Build history of the part. All positions in model axes, mm. Face numbers are marked on the shaded views. A direction names the side the tool comes from. Round coordinates to 2 decimals unless told otherwise and drop trailing zeros. Order: outer loops, then holes, each group sorted by start corner. A loop starts at its lowest first (then second) coordinate and runs counter-clockwise, first axis right, second up. Notation, with made-up numbers: (-14.75, -37) - (30.25, -37) arc R13 cw to (30.25, -14) - close; hole circle Ø8 at (74, 75.5). An arc over 180 degrees is marked (long way). Write each question's results on one line, items separated by ' | '. Start each with the question number.
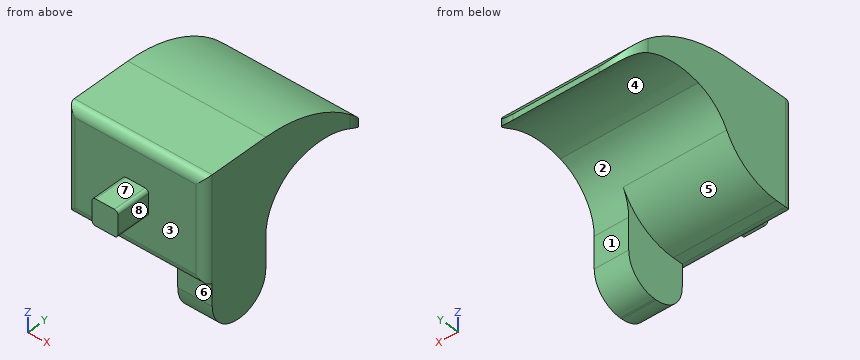
```python
from build123d import *

# Parameters (mm, degrees)
SKETCH1_W           = 80
SKETCH1_H           = 60
BOSS_EXTRUDE1_DEPTH = 40
SKETCH2_W           = 80
SKETCH2_H           = 40
BOSS_EXTRUDE2_DEPTH = 70
CUT_EXTRUDE1_REACH  = 141.284
FILLET4_R           = 31
FILLET6_R           = 5
FILLET7_R           = 15
SKETCH5_W           = 20
SKETCH5_H           = 35
BOSS_EXTRUDE4_DEPTH = 30
FILLET8_R           = 17
FILLET9_R           = 37
SKETCH6_W           = 15
SKETCH6_H           = 15
BOSS_EXTRUDE5_DEPTH = 20
FILLET10_R          = 2


with BuildPart() as part:
    # Sketch1 → Boss-Extrude1 (new body)
    with BuildSketch(Plane(origin=(0, 0, 0), x_dir=(1, 0, 0), z_dir=(0, 1, 0))):
        Rectangle(SKETCH1_W, SKETCH1_H)
    extrude(amount=BOSS_EXTRUDE1_DEPTH)

    # Sketch2 → Boss-Extrude2 (add)
    with BuildSketch(Plane(origin=(0, 40, 0), x_dir=(1, 0, 0), z_dir=(0, 1, 0))):
        with Locations((0, -10)):
            Rectangle(SKETCH2_W, SKETCH2_H)
    extrude(amount=BOSS_EXTRUDE2_DEPTH)

    # Sketch3 → Cut-Extrude1 (cut, up to next)
    with BuildSketch(Plane(origin=(40, 0, 0), x_dir=(0, 0, -1), z_dir=(1, 0, 0)), mode=Mode.PRIVATE) as cut_extrude1_sk1:
        with BuildLine():
            ThreePointArc((10, 110), (-6.715728753, 75), (10, 40))
            Line((10, 40), (10, 110))
        make_face()
    cut_extrude1_tool1 = extrude(cut_extrude1_sk1.sketch, amount=-CUT_EXTRUDE1_REACH, mode=Mode.PRIVATE) & part.part
    # Sketch3 → Cut-Extrude1 (cut, up to next)
    with BuildSketch(Plane(origin=(40, 0, 0), x_dir=(0, 0, -1), z_dir=(1, 0, 0)), mode=Mode.PRIVATE) as cut_extrude1_sk2:
        with BuildLine():
            ThreePointArc((-30, 40), (-20.28517386, 79.505502482), (6.643401936, 110))
            Line((6.643401936, 110), (-30, 110))
            Line((-30, 110), (-30, 40))
        make_face()
    cut_extrude1_tool2 = extrude(cut_extrude1_sk2.sketch, amount=-CUT_EXTRUDE1_REACH, mode=Mode.PRIVATE) & part.part
    add(cut_extrude1_tool1.solids().sort_by_distance((40, 75, -3.194337))[0], mode=Mode.SUBTRACT)
    add(cut_extrude1_tool2.solids().sort_by_distance((40, 93.341036, 19.578223))[0], mode=Mode.SUBTRACT)

    # Fillet4
    fillet4_edges = [part.edges().sort_by_distance(p)[0] for p in [
        (0, 40, -10),
    ]]
    fillet(fillet4_edges, radius=FILLET4_R)

    # Fillet6
    fillet6_edges = [part.edges().sort_by_distance(p)[0] for p in [
        (0, 0, -30),
        (40, 0, 0),
        (0, 0, 30),
        (-40, 0, 0),
    ]]
    fillet(fillet6_edges, radius=FILLET6_R)

    # Fillet7
    # the kernel refuses this fillet: 15 mm, written as the material it takes off along each edge
    with BuildSketch(Plane(origin=(-40, 110, -47.5), x_dir=(1, 0, 0), z_dir=(0, 0, 1))) as fillet7_piece_1:
        with BuildLine():
            CenterArc((FILLET7_R, -FILLET7_R), FILLET7_R, 90, 90)
            Line((0, -FILLET7_R), (0, 0))
            Line((0, 0), (FILLET7_R, 0))
        make_face()
    extrude(amount=78.356598064, mode=Mode.SUBTRACT)
    with BuildSketch(Plane(origin=(40, 110, 30.856598064), x_dir=(0, -1, 0), z_dir=(0, 0, -1))) as fillet7_piece_2:
        with BuildLine():
            CenterArc((FILLET7_R, FILLET7_R), FILLET7_R, 180, 90)
            Line((0, FILLET7_R), (0, 0))
            Line((0, 0), (FILLET7_R, 0))
        make_face()
    extrude(amount=78.356598064, mode=Mode.SUBTRACT)

    # Sketch5 → Boss-Extrude4 (add)
    with BuildSketch(Plane(origin=(0, 0, -30), x_dir=(-1, 0, 0), z_dir=(0, 0, -1))):
        with Locations((-30, 22.5)):
            Rectangle(SKETCH5_W, SKETCH5_H)
    extrude(amount=BOSS_EXTRUDE4_DEPTH)

    # Fillet8
    fillet8_edges = [part.edges().sort_by_distance(p)[0] for p in [
        (30, 5, -60),
        (30, 40, -60),
    ]]
    fillet(fillet8_edges, radius=FILLET8_R)

    # Fillet9
    # the kernel refuses this fillet: 37 mm, written as the material it takes off along each edge
    with BuildSketch(Plane(origin=(20, 40, -30), x_dir=(0, 0.18084372085202682, 0.9835118446812903), z_dir=(-1, 0, 0))) as fillet9_piece_1:
        with BuildLine():
            CenterArc((31.132759532, -35.282188472), FILLET9_R, 107.527471669, 62.053620325)
            Line((-5.257178722, -28.5909708), (-8.896172547, -27.921849033))
            Line((-8.896172547, -27.921849033), (-3.638993825, 0.669121767))
            Line((-3.638993825, 0.669121767), (0.669121767, 3.638993825))
            ThreePointArc((0.669121767, 3.638993825), (5.716638919, 2.710879143), (18.875423616, 3.528218847))
            Line((18.875423616, 3.528218847), (19.989726881, 0))
        make_face()
    extrude(amount=132.675715485, mode=Mode.SUBTRACT)

    # Sketch6 → Boss-Extrude5 (add)
    with BuildSketch(Plane.XZ):
        Rectangle(SKETCH6_W, SKETCH6_H)
    extrude(amount=BOSS_EXTRUDE5_DEPTH)

    # Fillet10
    fillet10_edges = [part.edges().sort_by_distance(p)[0] for p in [
        (-7.5, -10, 7.5),
        (-7.5, -10, -7.5),
        (7.5, -10, -7.5),
        (7.5, -10, 7.5),
    ]]
    fillet(fillet10_edges, radius=FILLET10_R)


solid = part.part
```
1. Cut at D-D (x = 22.5). List the corners of the cut face in (y, z), plus the area to 3 significant figures.
2. Cut at A-A (x = -4). List the corners of the cut face in (y, z), plus the area to 3 significant figures.
3. Cut at B-B (z = -21). List the corners of the cut face in (x, y).
4. 3-axis set-ups, long thin cutter, end or side, ignore diameter. For the marked faces 5, 6, 7 and 8: which of +Z, -Z, +X, -X, +Y, -Y reach the whole face in a straight line?
5. Mould opens along Y. For the marked faces 1, 2, 3 and 4 say: pulls with the +Y half, pulls with the -Y half, needs draft (parallel to the pull), parting line crosses it, or undercut.
6. Wall check: line 1 (Y direction, x = 36, z = -35); line 2 (Y direction, x = -25, z = 3); line 3 (Z direction, x = 4.5, y = 8). Give the ranges that are in metal, low to high. Write a range as from..to.
7. Flat gauge pins, fed straight in: pin 1 Ø12 at (y, z) = (-14.5, 1.5) entering from -X; pin 2 Ø3.5 at (x, y) = (-1, -11.5) entering from +Z; pin 3 Ø12 at (x, y) = (0.5, -6.5) entering from -Z; pin 4 Ø1 at (x, z) = (-8, -31.5) entering from -Y. Where does each tip first touch, or does it go through?
8. Cut at C-C (y = 6.5). List the corners of the cut face in (x, z), plus the area to 3 significant figures.
A:
1) outline: (0, -25) arc R5 ccw to (5, -30) - (5, -43) arc R17 ccw to (22, -60) - (23, -60) arc R17 ccw to (40, -43) - (40, -24.87) arc R31 cw to (62.14, 4.84) arc R45 cw to (110, -10) - (110, -6.64) arc R85.18 ccw to (40, 30) - (5, 30) arc R5 ccw to (0, 25) - close | area: 4,580 mm^2
2) outline: (-20, -7.5) - (0, -7.5) - (0, -25) arc R5 ccw to (5, -30) - (10.93, -30) arc R37 ccw to (43.62, -10.34) arc R31 cw to (62.14, 4.84) arc R45 cw to (110, -10) - (110, -6.64) arc R85.18 ccw to (40, 30) - (5, 30) arc R5 ccw to (0, 25) - (0, 7.5) - (-20, 7.5) - close | area: 3,820 mm^2
3) outline: (-40, 5) arc R5 ccw to (-35, 0) - (35, 0) arc R5 ccw to (40, 5) - (40, 40.24) - (20, 40.24) - (20, 35.12) - (-40, 35.12) - close
4) face 5: -Z, -X, +Y | face 6: -Z, +X, -X, -Y | face 7: +Z, +X, -X, -Y | face 8: +Z, -Z, +X, -Y
5) face 1: pulls with the +Y half | face 2: undercut | face 3: pulls with the -Y half | face 4: undercut
6) line 1: y = 5..40 | line 2: y = 0..57.42, 92.91..102.22 | line 3: z = -30..30
7) pin 1: stops at x = -7.5 | pin 2: stops at z = 7.5 | pin 3: stops at z = -7.5 | pin 4: passes through
8) outline: (-40, -30) - (20, -30) - (20, -49.98) - (40, -49.98) - (40, 30) - (-40, 30) - close | area: 5,200 mm^2
